from build123d import *

# Parameters (mm, degrees)
SKETCH_1_W          = 125
SKETCH_1_H          = 40
EXTRUDE_1_DEPTH     = 15
SKETCH_2_R          = 8.9
SKETCH_2_R_2        = 4.5
SKETCH_2_R_3        = 13.3
CUT_EXTRUDE_1_DEPTH = 133.098448136
CHAMFER_1_SIZE      = 1
CHAMFER_2_SIZE      = 1
FILLET_1_R          = 1
SKETCH_3_W          = 40
SKETCH_3_H          = 61.182970239
CUT_EXTRUDE_2_DEPTH = 133.098448148
SKETCH_5_W          = 5
SKETCH_5_H          = 48.384785396
CUT_EXTRUDE_3_DEPTH = 133.098448148


with BuildPart() as part:
    # 草圖1 → 填料-伸長1 (new body)
    with BuildSketch(Plane(origin=(0, 0, 0), x_dir=(1, 0, 0), z_dir=(0, 1, 0))):
        with Locations((62.5, 20)):
            Rectangle(SKETCH_1_W, SKETCH_1_H)
    extrude(amount=EXTRUDE_1_DEPTH)

    # 草圖2 → 除料-伸長1 (cut, through all)
    with BuildSketch(Plane(origin=(0, 15, 0), x_dir=(1, 0, 0), z_dir=(0, 1, 0))):
        with Locations(Location((18.526668527, 20, 0), (0, 0, 270))):
            Circle(SKETCH_2_R)
        with Locations(Location((106.526668527, 20, 0), (0, 0, 270))):
            Circle(SKETCH_2_R_2)
        with Locations(Location((62.526668527, 20, 0), (0, 0, 270))):
            Circle(SKETCH_2_R_3)
    extrude(amount=-CUT_EXTRUDE_1_DEPTH, mode=Mode.SUBTRACT)

    # 導角1
    chamfer_1_edges = [part.edges().sort_by_distance(p)[0] for p in [
        (18.526668527, 15, -28.9),
    ]]
    chamfer(chamfer_1_edges, length=CHAMFER_1_SIZE)

    # 導角2
    chamfer_2_edges = [part.edges().sort_by_distance(p)[0] for p in [
        (18.526668527, 0, -28.9),
    ]]
    chamfer(chamfer_2_edges, length=CHAMFER_2_SIZE)

    # 圓角1
    fillet_1_edges = [part.edges().sort_by_distance(p)[0] for p in [
        (106.526668527, 0, -24.5),
        (106.526668527, 15, -24.5),
        (62.526668527, 0, -33.3),
        (62.526668527, 15, -33.3),
    ]]
    fillet(fillet_1_edges, radius=FILLET_1_R)

    # 草圖3 → 除料-伸長2 (cut, through all)
    with BuildSketch(Plane(origin=(0, 15, 0), x_dir=(1, 0, 0), z_dir=(0, 1, 0))):
        with Locations((20, 30.59148512)):
            Rectangle(SKETCH_3_W, SKETCH_3_H)
    extrude(amount=-CUT_EXTRUDE_2_DEPTH, mode=Mode.SUBTRACT)

    # 草圖5 → 除料-伸長3 (cut, through all)
    with BuildSketch(Plane(origin=(0, 15, 0), x_dir=(1, 0, 0), z_dir=(0, 1, 0))):
        with Locations((122.5, 24.192392698)):
            Rectangle(SKETCH_5_W, SKETCH_5_H)
    extrude(amount=-CUT_EXTRUDE_3_DEPTH, mode=Mode.SUBTRACT)


solid = part.part
Read the model definition and answer for the solid it produces. Units are mm, in the model's axes. Give positions to 0.01 mm unless a question says otherwise; leave off trailing zeros. Loops run counter-clockwise (first coordinate to the right, second up) from the corner with the lowest first, then second, coordinate; pieces in that order, holes last. Notation, with made-up numbers: (41, 67.25) - (60, 67.25) arc R25 cw to (60, 103.25) - close; hole circle Ø11 at (-2.75, -33). An arc over 180 degrees is marked (long way). Answer as CSV lines item,"result". Start each with the question number.
1) Straight lines are drawn through the part: L1, parallel to X at y = 10.75, z = -20; L2, parallel to Z at x = 67, y = 6.75; L3, parallel to X at y = 7.25, z = -19. For each, find the intervals that lie inside material, in ascending order. Write a range as from..to.
2) Find section A-A (z = -20). Write down the section's boundary in (x, y), then the cut area to 3 significant figures.
3) Find section B-B (y = 2.25). Write down the section's boundary in (x, z).
4) Determine the mould class of faces 1 (the face through (40, 8, -20)), 2 (the face through (79, 7, 0)), 3 (the face through (57.433, 7.591, -7.714)) for opening direction X: released by +X, released by -X, zero draft, split by the parting line, or undercut.
Findings below:
1,L1,"40..49.23, 75.83..102.03, 111.03..120"
1,L2,"-40..-32.53, -7.47..0"
1,L3,"40..49.26, 75.79..102.14, 110.91..120"
2,outline,"(40, 0) - (48.23, 0) arc R1 ccw to (49.23, 1) - (49.23, 14) arc R1 ccw to (48.23, 15) - (40, 15) - close; (75.83, 1) arc R1 ccw to (76.83, 0) - (101.03, 0) arc R1 ccw to (102.03, 1) - (102.03, 14) arc R1 ccw to (101.03, 15) - (76.83, 15) arc R1 ccw to (75.83, 14) - close; (111.03, 1) arc R1 ccw to (112.03, 0) - (120, 0) - (120, 15) - (112.03, 15) arc R1 ccw to (111.03, 14) - close"
2,area,"664 mm^2"
3,outline,"(40, -40) - (120, -40) - (120, 0) - (40, 0) - close; hole circle Ø26.6 at (62.53, -20); hole circle Ø9 at (106.53, -20)"
4,face 1,"released by -X"
4,face 2,"zero draft"
4,face 3,"undercut"
